Autodesk Inventor part; units mm, degrees
ref_plane "YZ Plane" through (0, 0, 0) normal (1, 0, 0) x (0, 1, 0)
ref_plane "XZ Plane" through (0, 0, 0) normal (0, 1, 0) x (-1, 0, 0)
ref_plane "XY Plane" through (0, 0, 0) normal (0, 0, 1) x (1, 0, 0)
sketch "スケッチ1" plane through (0, 0, 0) normal (0, 0, 1) x (1, 0, 0)
  line L0 (0, 0) -> (45, 15)
  line L1 (45, 15) -> (75, 15)
  line L2 (75, 15) -> (75, 10)
  line L3 (75, 10) -> (45.8114, 10)
  line L4 (45.8114, 10) -> (15.8114, 0)
  line L5 (15.8114, 0) -> (0, 0)
  dimension "d0" = 15
  dimension "d1" = 5
  dimension "d2" = 5
  dimension "d21" = 30
  dimension "d27" = 30
extrude "押し出し1" add sketch "スケッチ1" along normal blind 120
sketch "スケッチ3" plane through (45, 15, 0) normal (0, 1, 0) x (1, 0, 0)
  line L0 (30, 0) -> (30, -120)
  line L1 (30, 0) -> (0, 0)
  line L2 (30, -120) -> (0, -120)
  point P0 (-45, 0)
  point P1 (15, -7)
  point P2 (30, -80)
  point P3 (15, -113)
  point P4 (15, -120)
  dimension "d12" = 15
  dimension "d13" = 7
  dimension "d23" = 106
hole "穴1" at (60, 15, 7) at (60, 15, 113) direction (0, -1, 0) diameter 3.2 depth 10 tip angle 118
properties part number "排出スロープ"
Read the model definition and answer for the solid it produces. Units are mm, in the model's axes. Coordinates: 2 decimals unless noted, no trailing zeros. Write each loop counter-clockwise with the first axis right and the second up, starting at its lowest first coordinate (ties: lowest second). Pieces come first, ordered by that corner, then holes. Notation, with made-up numbers: (40.5, 64.25) - (75.5, 64.25) arc R21 ccw to (75.5, 83.25) - close; hole circle Ø9 at (-28.5, -12). An arc over 180 degrees is marked (long way). One line per question, with ' | ' between items.
Q1. Find section A-A, the plane x = 60. Write down the section's boundary in (y, z).
Result set:
outline: (10, 0) - (15, 0) - (15, 5.4) - (10, 5.4) - close; (10, 8.6) - (15, 8.6) - (15, 111.4) - (10, 111.4) - close; (10, 114.6) - (15, 114.6) - (15, 120) - (10, 120) - close
Q2. Find section B-B, the plane z = 113. Write down the section's boundary in (x, y), plus the area to 3 significant figures.
Result set:
outline: (0, 0) - (15.81, 0) - (45.81, 10) - (58.4, 10) - (58.4, 15) - (45, 15) - close; (61.6, 10) - (75, 10) - (75, 15) - (61.6, 15) - close | area: 330 mm^2
Q3. Each of these flat-tipped pins is pushed along its axis until it touches: P1, Ø1.9, axis at x = 60, z = 7, coming from the +Y side; P2, Ø8, axis at x = 18.5, z = 89.5, coming from the +Y side; P3, Ø1, axis at x = 28, z = 28.5, coming from the -Y side; P4, Ø5, axis at x = 60, z = 113, coming from the -Y side. Where does it stop, or does it pass through?
Result set:
P1: through | P2: y = 7.5 | P3: y = 3.9 | P4: y = 10
Q4. Find section D-D, the plane z = 66.5. Write down the section's boundary in (x, y), plus the area to 3 significant figures.
Result set:
outline: (0, 0) - (15.81, 0) - (45.81, 10) - (75, 10) - (75, 15) - (45, 15) - close | area: 346 mm^2
Q5. Find section C-C, the plane y = 13.75. Write down the section's boundary in (x, z), plus the area to 3 significant figures.
Result set:
outline: (41.25, 0) - (75, 0) - (75, 120) - (41.25, 120) - close; hole circle Ø3.2 at (60, 7); hole circle Ø3.2 at (60, 113) | area: 4,030 mm^2
Q6. Determine the mould class of faces 1 (the cylindrical face through (59.519, 12.465, 114.526)), 2 (the cylindrical face through (58.414, 12.465, 6.792)), 3 (the flat face through (40, 9, 0)), 4 (the flat face through (61, 10, 59)) for opening direction Z: +Z half, -Z half, draft (parallel to the pull), parting line (faces both ways), or undercut.
Result set:
face 1: undercut | face 2: undercut | face 3: -Z half | face 4: draft
Q7. Consider L1, parallel to Z at x = 60, y = 12.9; L2, parallel to Y at x = 47, z = 94; L3, parallel to Y at x = 41, z = 31.5. Determine where each line is inside the solid, lowest interval first. Write a range as [from, to].
Result set:
L1: [0, 5.4], [8.6, 111.4], [114.6, 120] | L2: [10, 15] | L3: [8.4, 13.67]
